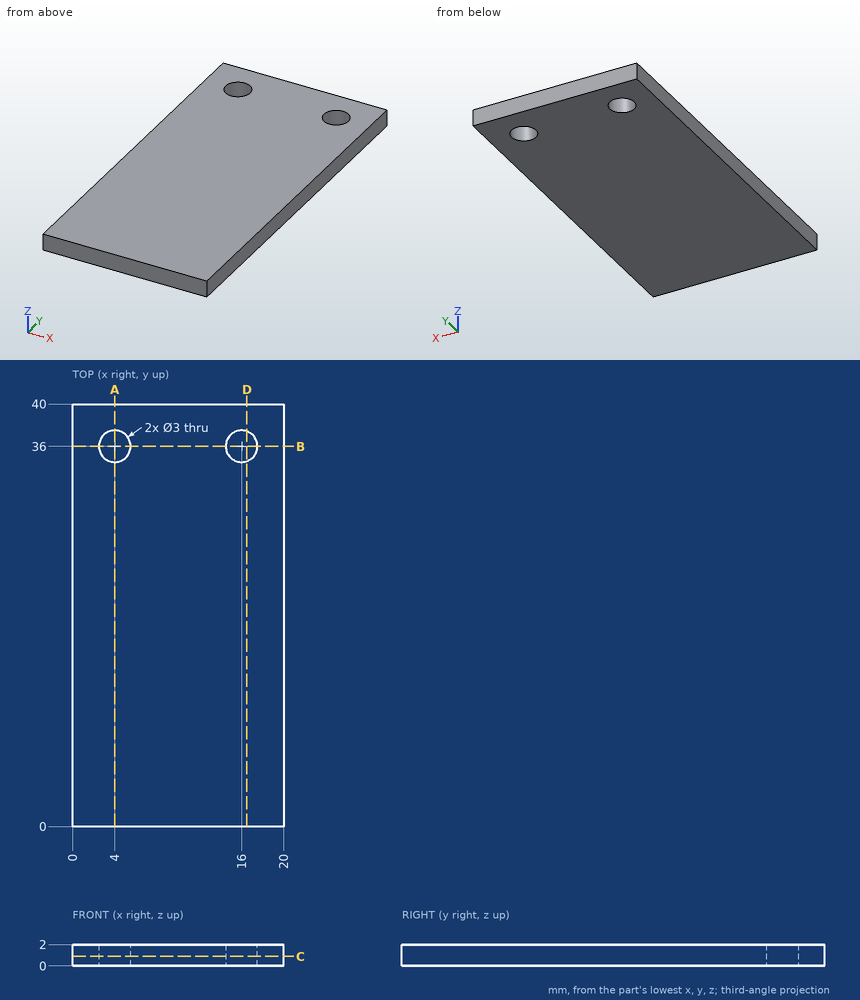
Verification items for this drawing (mm, ordinates from the low corner). Give positions to 0.01 mm unless a question says otherwise; leave off trailing zeros. Write each loop counter-clockwise with the first axis right and the second up, starting at its lowest first coordinate (ties: lowest second). Pieces come first, ordered by that corner, then holes. Notation, with made-up numbers: (-6, 76.5) -> (41, 76.5) arc R17 cw to (41, 80.5) -> close; hole circle Ø8 at (13, 54.5). An arc over 180 degrees is marked (long way). Use CSV: the item, a comma, the result in double quotes.
(1) Sectioned sample at C-C (z = 0.9). Record the cut outline in (x, y), plus the area to 3 significant figures.
Derived:
outline,"(0, 0) -> (20, 0) -> (20, 40) -> (0, 40) -> close; hole circle Ø3 at (4, 36); hole circle Ø3 at (16, 36)"
area,"786 mm^2"
(2) Go/stop test with a flat-tipped pin: pin 1 (2.5 mm diameter, centred on x = 16, y = 36, fed in from -Z) (3 decimals). Record where the tip stops, or that it passes through.
Derived:
pin 1,"passes through"
(3) Sectioned sample at D-D (x = 16.5). Record the cut outline in (y, z).
Derived:
outline,"(0, 0) -> (34.59, 0) -> (34.59, 2) -> (0, 2) -> close; (37.41, 0) -> (40, 0) -> (40, 2) -> (37.41, 2) -> close"
(4) Material ranges on L1, parallel to Y at x = 4, z = 0.7; L2, parallel to Y at x = 17, z = 0.85, recorded low to high.
Derived:
L1,"y = 0 to 34.5, 37.5 to 40"
L2,"y = 0 to 34.88, 37.12 to 40"
(5) Sectioned sample at A-A (x = 4). Record the cut outline in (y, z), plus the area to 3 significant figures.
Derived:
outline,"(0, 0) -> (34.5, 0) -> (34.5, 2) -> (0, 2) -> close; (37.5, 0) -> (40, 0) -> (40, 2) -> (37.5, 2) -> close"
area,"74.0 mm^2"
(6) Sectioned sample at B-B (y = 36). Record the cut outline in (x, z).
Derived:
outline,"(0, 0) -> (2.5, 0) -> (2.5, 2) -> (0, 2) -> close; (5.5, 0) -> (14.5, 0) -> (14.5, 2) -> (5.5, 2) -> close; (17.5, 0) -> (20, 0) -> (20, 2) -> (17.5, 2) -> close"
